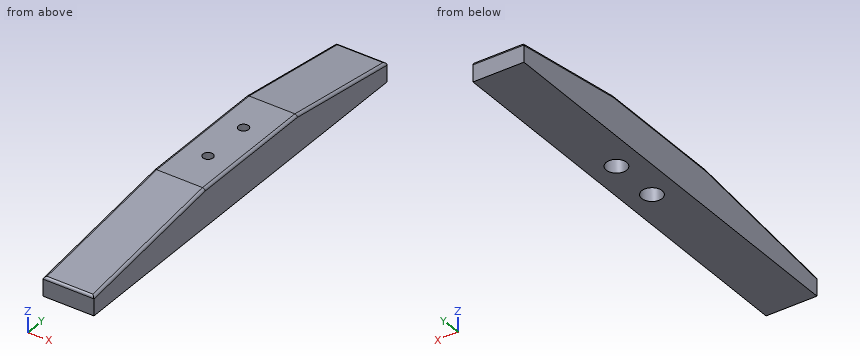
from build123d import *

# Parameters (mm, degrees)
PAD_DEPTH       = 20
SKETCH001_R     = 2
POCKET_DEPTH    = 15.001
SKETCH002_R     = 4
POCKET001_DEPTH = 8
FILLET_R        = 1


with BuildPart() as part:
    # Sketch (on YZ_Plane of Origin) → Pad (new body)
    with BuildSketch(Plane.YZ):
        Polygon((-84.432856, 0), (80.567144, 0), (80.567144, 7.5), (30.15051, 15), (-21.84949, 15), (-84.432856, 7.5), align=None)
    extrude(amount=PAD_DEPTH)

    # Sketch001 (on Face4 of Pad) → Pocket (cut, through all)
    with BuildSketch(Plane.XY.offset(15)):
        with Locations((10, 14.15051)):
            Circle(SKETCH001_R)
        with Locations((10, -5.84949)):
            Circle(SKETCH001_R)
    extrude(amount=-POCKET_DEPTH, mode=Mode.SUBTRACT)

    # Sketch002 (on Face1 of Pocket) → Pocket001 (cut)
    with BuildSketch(Plane(origin=(0, 0, 0), x_dir=(1, 0, 0), z_dir=(0, 0, -1))):
        with Locations((10, 5.84949)):
            Circle(SKETCH002_R)
        with Locations((10, -14.15051)):
            Circle(SKETCH002_R)
    extrude(amount=-POCKET001_DEPTH, mode=Mode.SUBTRACT)

    # Fillet
    fillet_edges = [part.edges().sort_by_distance(p)[0] for p in [
        (10, -84.432856, 7.5),
        (0, -53.141173, 11.25),
        (20, -53.141173, 11.25),
        (20, 4.15051, 15),
        (0, 4.15051, 15),
        (0, 55.358827, 11.25),
        (20, 55.358827, 11.25),
        (10, 80.567144, 7.5),
    ]]
    fillet(fillet_edges, radius=FILLET_R)


solid = part.part
Build history of the part. All positions in model axes, mm. Give positions to 0.01 mm unless a question says otherwise; leave off trailing zeros. Loops run counter-clockwise (first coordinate to the right, second up) from the corner with the lowest first, then second, coordinate; pieces in that order, holes last. Notation, with made-up numbers: (-7, 26) - (10, 26) arc R26 ccw to (10, 48) - close; hole circle Ø2 at (-6, -5.75). An arc over 180 degrees is marked (long way). Write item = value, one per line. Start each with the question number.
1) Probe probe 1 along Y at (x, z) = (10, 4.75); probe 2 along Y at (x, z) = (9.25, 6.25); probe 3 along X at (y, z) = (-5.5, 6.75). List the from-to ranges inside material, lowest first. Write a range as from..to.
2) Drop flat-ended pins along their axis: pin 1 Ø2.5 at (x, y) = (10.5, 13.5) entering from -Z; pin 2 Ø10 at (x, y) = (8, -34) entering from +Z. Give the stop position or say it passes through.
3) Band-saw the part on A-A on x = 10. Give the cut face in (y, z).
4) Band-saw the part on B-B on x = 2.5. Give the cut face in (y, z).
5) Band-saw the part on C-C on z = 4. Give the cut face in (x, y).
Final values:
q1.probe_1 = -84.43..-9.85, -1.85..10.15, 18.15..80.57
q1.probe_2 = -84.43..-9.78, -1.92..10.22, 18.08..80.57
q1.probe_3 = 0..6.02, 13.98..20
q2.pin_1 = 8
q2.pin_2 = 14.14
q3.outline = (-84.43, 0) - (-9.85, 0) - (-9.85, 8) - (-7.85, 8) - (-7.85, 15) - (-21.85, 15) - (-83.55, 7.61) arc R1 ccw to (-84.43, 6.61) - close; (-3.85, 8) - (-1.85, 8) - (-1.85, 0) - (10.15, 0) - (10.15, 8) - (12.15, 8) - (12.15, 15) - (-3.85, 15) - close; (16.15, 8) - (18.15, 8) - (18.15, 0) - (80.57, 0) - (80.57, 6.64) arc R1 ccw to (79.71, 7.63) - (30.15, 15) - (16.15, 15) - close
q4.outline = (-84.43, 0) - (80.57, 0) - (80.57, 6.64) arc R1 ccw to (79.71, 7.63) - (30.15, 15) - (-21.85, 15) - (-83.55, 7.61) arc R1 ccw to (-84.43, 6.61) - close
q5.outline = (0, -84.43) - (20, -84.43) - (20, 80.57) - (0, 80.57) - close; hole circle Ø8 at (10, -5.85); hole circle Ø8 at (10, 14.15)
